```python
from build123d import *

# Parameters (mm, degrees)
SKETCH_2_R      = 1.6
EXTRUDE_1_DEPTH = 2


with BuildPart() as part:
    # 草图2 → 凸台-拉伸1 (new body)
    with BuildSketch(Plane(origin=(0, 0, 0), x_dir=(1, 0, 0), z_dir=(0, 1, 0))):
        with BuildLine():
            Line((-8, 4), (0, 4))
            ThreePointArc((0, 4), (15.110526316, 2.840032678), (29.866957344, -0.612686981))
            ThreePointArc((29.866957344, -0.612686981), (32.473840401, -5.633061541), (27.453465841, -8.239944598))
            ThreePointArc((27.453465841, -8.239944598), (13.889473684, -5.066232589), (0, -4))
            Line((0, -4), (-8, -4))
            ThreePointArc((-8, -4), (-12, 0), (-8, 4))
        make_face()
        with Locations((-8, 0)):
            Circle(SKETCH_2_R, mode=Mode.SUBTRACT)
        with BuildLine():
            ThreePointArc((29.142909893, -2.900864266), (14.744210526, 0.468153098), (0, 1.6))
            ThreePointArc((0, 1.6), (-1.6, 0), (0, -1.6))
            ThreePointArc((0, -1.6), (14.255789474, -2.694353009), (28.177513292, -5.951767313))
            ThreePointArc((28.177513292, -5.951767313), (30.185663116, -4.90901409), (29.142909893, -2.900864266))
        make_face(mode=Mode.SUBTRACT)
    extrude(amount=EXTRUDE_1_DEPTH)


solid = part.part
```
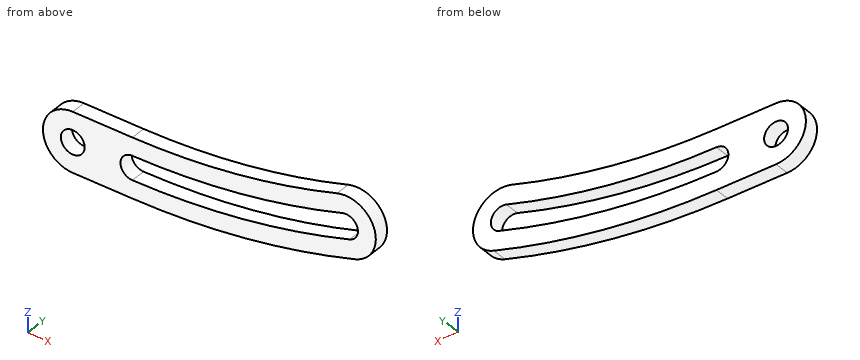
Work out the finished part from the listing and answer in its coordinate system (mm). Give positions to 0.01 mm unless a question says otherwise; leave off trailing zeros. Loops run counter-clockwise (first coordinate to the right, second up) from the corner with the lowest first, then second, coordinate; pieces in that order, holes last. Notation, with made-up numbers: (50, 62.5) -> (68, 62.5) arc R25 cw to (68, 101.5) -> close; hole circle Ø6 at (-26, 77.25). An arc over 180 degrees is marked (long way). One line per question, with ' | ' between items. Start each with the question number.
1) Each of these flat-tipped pins is pushed along its axis until it touches: pin 1 (4 mm diameter, centred on x = -3, z = -1, fed in from -Y); pin 2 (0.6 mm diameter, centred on x = -3, y = 1, fed in from +Z). Where does it stop, or does it pass through?
2) Section C-C, the plane x = -7 is taken. Determine the outline of the cut face in (y, z).
3) Straight lines are drawn through the part: L1, parallel to Z at x = -8, y = 1.5; L2, parallel to Z at x = 12, y = 0.95; L3, parallel to Z at x = -3, y = 0.3. For each, find the intervals that lie inside material, in ascending order.
4) Section A-A, the plane y = 1.6 is taken. Determine the outline of the cut face in (x, z), then the cut area to 3 significant figures.
5) Section D-D, the plane z = -0.5 is taken. Determine the outline of the cut face in (x, y).
Resolved:
1) pin 1: y = 0 | pin 2: z = 4
2) outline: (0, -4) -> (2, -4) -> (2, -1.25) -> (0, -1.25) -> close; (0, 1.25) -> (2, 1.25) -> (2, 4) -> (0, 4) -> close
3) L1: -4 to -1.6, 1.6 to 4 | L2: -3.27 to -0.85, 2.37 to 4.79 | L3: -4 to 4
4) outline: (-8, -4) -> (0, -4) arc R99 ccw to (29.87, 0.61) arc R4 ccw to (27.45, 8.24) arc R91 cw to (0, 4) -> (-8, 4) arc R4 ccw to start; hole circle Ø3.2 at (-8, 0); hole (0, -1.6) arc R96.6 ccw to (29.14, 2.9) arc R1.6 ccw to (28.18, 5.95) arc R93.4 cw to (0, 1.6) arc R1.6 ccw to start | area: 238 mm2
5) outline: (-11.97, 0) -> (-9.52, 0) -> (-9.52, 2) -> (-11.97, 2) -> close; (-6.48, 0) -> (-1.52, 0) -> (-1.52, 2) -> (-6.48, 2) -> close; (14.54, 0) -> (26.09, 0) -> (26.09, 2) -> (14.54, 2) -> close
